Autodesk Inventor part; units mm, degrees
ref_plane "YZ Plane" through (0, 0, 0) normal (1, 0, 0) x (0, 1, 0)
ref_plane "XZ Plane" through (0, 0, 0) normal (0, 1, 0) x (-1, 0, 0)
ref_plane "XY Plane" through (0, 0, 0) normal (0, 0, 1) x (1, 0, 0)
sketch "Sketch1" plane through (0, 0, 0) normal (0, 0, 1) x (1, 0, 0)
  line L0 (10.9384, 8.2044) -> (170.9384, 8.2044)
  line L1 (170.9384, 8.2044) -> (170.9384, 98.2044)
  line L2 (10.9384, 98.2044) -> (10.9384, 8.2044)
  line L3 (10.9384, 98.2044) -> (60.9384, 158.2044)
  line L4 (60.9384, 158.2044) -> (120.9384, 158.2044)
  line L5 (120.9384, 158.2044) -> (170.9384, 98.2044)
  dimension "d0" = 160
  dimension "d4" = 60
  dimension "d5" = 50
  dimension "d6" = 90
  dimension "d7" = 90
  dimension "d8" = 150
extrude "Extrusion1" add sketch "Sketch1" along normal blind 1.8974
sketch "Sketch2" plane through (0, 0, 1.8974) normal (0, 0, 1) x (1, 0, 0)
  line L0 (10.9384, 8.2044) -> (10.9384, 98.2044)
  line L1 (170.9384, 8.2044) -> (10.9384, 8.2044)
  circle A0 centre (20.9384, 20.9044) radius 3.5685
  circle A1 centre (20.9384, 85.5044) radius 2.5
  dimension "d11" = 7.137
  dimension "d12" = 12.7
  dimension "d13" = 10
  dimension "d14" = 10
  dimension "d15" = 64.6
  dimension "d16" = 5
extrude "Extrusion2" cut sketch "Sketch2" against normal through all
pattern_linear "Rectangular Pattern1" count 2 spacing 140 along (1, 0, 0) of "Extrusion2"
sketch "Sketch3" plane through (0, 0, 1.8974) normal (0, 0, 1) x (1, 0, 0)
  line L0 (10.9384, 8.2044) -> (10.9384, 98.2044)
  line L1 (170.9384, 8.2044) -> (10.9384, 8.2044)
  circle A0 centre (90.9384, 85.5044) radius 6.5
  circle A1 centre (75.4444, 70.0104) radius 1.5
  circle A2 centre (106.4324, 70.0104) radius 1.5
  circle A3 centre (75.4444, 100.9984) radius 1.5
  circle A4 centre (106.4324, 100.9984) radius 1.5
  dimension "d22" = 13
  dimension "d23" = 80
  dimension "d24" = 77.3
  dimension "d27" = 3
  dimension "d28" = 61.806
  dimension "d29" = 64.506
  dimension "d30" = 3
  dimension "d31" = 61.806
  dimension "d32" = 95.494
  dimension "d33" = 3
  dimension "d34" = 3
  dimension "d35" = 64.506
  dimension "d36" = 92.794
  dimension "d37" = 92.794
  dimension "d38" = 95.494
extrude "Extrusion3" cut sketch "Sketch3" against normal through all
sketch "Sketch4" plane through (0, 0, 1.8974) normal (0, 0, 1) x (1, 0, 0)
  circle A0 centre (160.9384, 85.5044) radius 2.5
  circle A1 centre (20.9384, 85.5044) radius 2.5
  line L0 (10.9384, 8.2044) -> (10.9384, 98.2044)
  line L1 (170.9384, 98.2044) -> (170.9384, 8.2044)
  circle A2 centre (55.9384, 98.2044) radius 2.5
  circle A3 centre (135.9384, 98.2044) radius 2.5
  dimension "d39" = 45
  dimension "d40" = 12.7
  dimension "d41" = 5
  dimension "d42" = 35
  dimension "d43" = 12.7
  dimension "d44" = 5
extrude "Extrusion4" cut sketch "Sketch4" against normal through all contours A2 | A3
sketch "Sketch5" plane through (0, 0, 1.8974) normal (0, 0, 1) x (1, 0, 0)
  line L0 (60.9384, 158.2044) -> (120.9384, 158.2044)
  circle A0 centre (110.9384, 148.2044) radius 2.5
  circle A1 centre (110.9384, 128.2044) radius 2.5
  dimension "d47" = 10
  dimension "d48" = 10
  dimension "d49" = 20
  dimension "d50" = 10
  dimension "d51" = 5
  dimension "d52" = 5
extrude "Extrusion5" cut sketch "Sketch5" against normal through all
sketch "Sketch6" plane through (0, 0, 1.8974) normal (0, 0, 1) x (1, 0, 0)
  line L0 (10.9384, 8.2044) -> (10.9384, 98.2044)
  line L1 (170.9384, 8.2044) -> (10.9384, 8.2044)
  circle A0 centre (67.3264, 61.8746) radius 2.54
  dimension "d55" = 56.388
  dimension "d56" = 53.6702
  dimension "d57" = 5.08
extrude "Extrusion6" cut sketch "Sketch6" against normal through all
pattern_linear "Rectangular Pattern2" count 2 spacing 47.244 along (1, 0, 0) count 2 spacing 47.244 along (0, 1, 0) of "Extrusion6"
fillet "Fillet2" radius 3.175 6 edges at (120.9384, 158.2044, 0.9487) (60.9384, 158.2044, 0.9487) (170.9384, 98.2044, 0.9487) (170.9384, 8.2044, 0.9487) (10.9384, 98.2044, 0.9487) (10.9384, 8.2044, 0.9487)
sketch "Sketch7" plane through (0, 0, 0) normal (0, 0, -1) x (-1, 0, 0)
  line L0 (-10.9384, 97.0549) -> (-10.9384, 11.3794)
  line L1 (-170.9384, 11.3794) -> (-170.9384, 97.0549)
  line L2 (-14.1134, 8.2044) -> (-167.7634, 8.2044)
  circle A0 centre (-140.9384, 20.9044) radius 2.5
  circle A1 centre (-40.9384, 20.9044) radius 2.5
  dimension "d68" = 5
  dimension "d69" = 12.7
  dimension "d70" = 30
  dimension "d71" = 5
  dimension "d72" = 30
  dimension "d73" = 12.7
extrude "Extrusion7" cut sketch "Sketch7" against normal through all
ref_plane "Work Plane1" through (90.9384, 158.2044, 1.8974) normal (0, 0, 1) x (1, 0, 0)
ref_plane "Work Plane2" through (90.9384, 158.2044, 1.8974) normal (-1, 0, 0) x (0, 0, 1)
mirror "Mirror1" about plane through (90.9384, 158.2044, 1.8974) normal (-1, 0, 0) of "Extrusion5"
equation "\"d7\" = d6"
equation "\"d30\" = d27"
equation "\"d31\" = d28"
equation "\"d33\" = d27"
equation "\"d34\" = d27"
equation "\"d35\" = d29"
equation "\"d50\" = d48"
properties part number "SM-S01" material "Steel, Mild"
Model file for the job. Use its own axes, mm. Give positions to 0.01 mm unless a question says otherwise; leave off trailing zeros. Order: outer loops, then holes, each group sorted by start corner. A loop starts at its lowest first (then second) coordinate and runs counter-clockwise, first axis right, second up. Notation, with made-up numbers: (20.25, 86.5) - (37.25, 86.5) arc R13 ccw to (37.25, 104.5) - close; hole circle Ø5 at (31.25, -20.75). An arc over 180 degrees is marked (long way). Return JSON: item names as keys, results as strings.
1) Cut at A-A, the plane x = 91. Give the cut face in (y, z), plus the area to 3 significant figures.
Geometry says:
{"outline": "(8.2, 0) - (79, 0) - (79, 1.9) - (8.2, 1.9) - close; (92, 0) - (158.2, 0) - (158.2, 1.9) - (92, 1.9) - close", "area": "260 mm²"}
2) Probe line 1 (X direction, y = 62, z = 1.15); line 2 (Y direction, x = 67.5, z = 0.4); line 3 (X direction, y = 21, z = 1.3). List the from-to ranges inside material, lowest first. Write a range as from..to.
Geometry says:
{"line 1": "10.94..64.79, 69.86..112.03, 117.11..170.94", "line 2": "8.2..59.34, 64.41..106.58, 111.65..158.2", "line 3": "10.94..17.37, 24.51..38.44, 43.44..138.44, 143.44..157.37, 164.51..170.94"}
3) Cut at D-D, the plane y = 119. Give the cut face in (x, z), plus the area to 3 significant figures.
Geometry says:
{"outline": "(28.27, 0) - (153.61, 0) - (153.61, 1.9) - (28.27, 1.9) - close", "area": "238 mm²"}
4) Cut at C-C, the plane x = 50. Give the cut face in (y, z), plus the area to 3 significant figures.
Geometry says:
{"outline": "(8.2, 0) - (145.08, 0) - (145.08, 1.9) - (8.2, 1.9) - close", "area": "260 mm²"}
5) Flat gauge pins, fed straight in: P1, Ø2, axis at x = 61, y = 116, coming from the -Z side; P2, Ø4, axis at x = 114.57, y = 109.12, coming from the -Z side. Where does each tip first touch, or does it go through?
Geometry says:
{"P1": "z = 0", "P2": "through"}
6) Cut at B-B, the plane z = 0.95. Count the separate pieces of the cut face and the enclosed holes in it, plus the area to 3 significant figures.
Geometry says:
{"separate pieces": "1", "enclosed holes": "21", "area": "20,500 mm²"}
7) Pull direction X, two halves, no side cores. Call faces 1 (the flat face through (145.71, 128.48, 0.94)), 2 (the cylindrical face through (116.993, 62.638, 0.962)), 3 (the flat face through (90, 68, 0)): pulls with the +X half, pulls with the -X half, needs draft (parallel to the pull), parting line crosses it, or undercut.
Geometry says:
{"face 1": "pulls with the +X half", "face 2": "undercut", "face 3": "needs draft"}
